Work out the finished part from the listing and answer in its coordinate system (mm). A direction names the side the tool comes from. Round coordinates to 2 decimals unless told otherwise and drop trailing zeros. Loops run counter-clockwise (first coordinate to the right, second up) from the corner with the lowest first, then second, coordinate; pieces in that order, holes last.
Autodesk Inventor part; units mm, degrees
ref_plane "YZ Plane" through (0, 0, 0) normal (1, 0, 0) x (0, 1, 0)
ref_plane "XZ Plane" through (0, 0, 0) normal (0, 1, 0) x (-1, 0, 0)
ref_plane "XY Plane" through (0, 0, 0) normal (0, 0, 1) x (1, 0, 0)
sketch "Sketch1" plane through (0, 0, 0) normal (0, 1, 0) x (-1, 0, 0)
  line L0 (65, -64) -> (-65, -64)
  line L1 (-65, -64) -> (-65, -45)
  line L2 (-65, 52) -> (65, 52)
  line L3 (65, 52) -> (65, -15)
  line L4 (94, -45) -> (65, -45)
  line L5 (65, -45) -> (65, -15) construction
  line L6 (65, -15) -> (94, -15)
  line L7 (94, -15) -> (94, -45)
  line L8 (-65, -45) -> (-94, -45)
  line L9 (-94, -45) -> (-94, -15)
  line L10 (-94, -15) -> (-65, -15)
  line L11 (-65, -15) -> (-65, -30) construction
  line L12 (94, -30) -> (-94, -30) construction
  line L13 (65, -45) -> (65, -64)
  line L14 (65, -15) -> (65, -45) construction
  line L15 (-65, -45) -> (-65, -15) construction
  line L16 (-65, -30) -> (-65, -45) construction
  line L17 (-65, -15) -> (-65, 52)
  point P0 (0, 0)
  point P1 (0, 52)
  dimension "d0" = 116
  dimension "d1" = 130
  dimension "d2" = 52
  dimension "d3" = 30
  dimension "d4" = 30
  dimension "d5" = 188
extrude "Extrusion1" add sketch "Sketch1" along normal blind 20
fillet "Fillet1" radius 10 4 edges at (65, 10, 52) (-65, 10, 52) (-65, 10, -64) (65, 10, -64)
sketch "Sketch2" plane through (0, 20, 0) normal (0, 1, 0) x (1, 0, 0)
  line L0 (65, 15) -> (94, 15)
  line L1 (94, 15) -> (94, 45)
  line L2 (94, 45) -> (65, 45)
  line L3 (94, 15) -> (94, 45)
  line L4 (65, 15) -> (94, 15)
  line L5 (94, 45) -> (76, 45)
  line L6 (76, 45) -> (76, 15)
  line L7 (76, 15) -> (94, 15)
  line L8 (94, 15) -> (94, 45)
  point P0 (0, 0)
  dimension "d9" = 18
extrude "Extrusion2" add sketch "Sketch2" along normal blind 38
fillet "Fillet2" radius 15 2 edges at (85, 58, -15) (85, 58, -45)
mirror "Mirror1" about plane through (0, 0, 0) normal (1, 0, 0) of "Extrusion2", "Fillet2"
sketch "Sketch3" plane through (94, 0, -15) normal (1, 0, 0) x (0, 0, -1)
  arc A0 (30, 43) -> (0, 43) centre (15, 43) ccw
  point P0 (-15, 0)
hole "Hole1" at (94, 43, -30) direction (-1, 0, 0) diameter 16 end through all
sketch "Sketch4" plane through (0, 20, 0) normal (0, 1, 0) x (1, 0, 0)
  line L0 (-55, -52) -> (55, -52)
  arc A0 (0, 24.1868) -> (0, -24.1868) centre (-28, 0) ccw
  line L1 (55, 64) -> (-55, 64)
  line L2 (0, 64) -> (0, -52) construction
  arc A1 (0, -24.1868) -> (0, 24.1868) centre (28, 0) ccw
  point P0 (0, 0)
  dimension "d20" = 74
  dimension "d21" = 56
extrude "Extrusion3" add sketch "Sketch4" along normal blind 6
sketch "Sketch5" plane through (0, 26, 0) normal (0, 1, 0) x (1, 0, 0)
  arc A0 (0, 24.1868) -> (0, -24.1868) centre (-28, 0) ccw
  point P0 (0, 0)
hole "Hole2" at (-28, 26, 0) direction (0, -1, 0) diameter 46 depth 15
sketch "Sketch6" plane through (0, 26, 0) normal (0, 1, 0) x (1, 0, 0)
  arc A0 (0, -24.1868) -> (0, 24.1868) centre (28, 0) ccw
  point P0 (0, 0)
  point P1 (28, 0)
hole "Hole3" at (28, 26, 0) direction (0, -1, 0) diameter 46 depth 15
sketch "Sketch7" plane through (65, 0, -15) normal (1, 0, 0) x (0, 0, -1)
  line L0 (-57, 0) -> (0, 0)
  line L1 (0, 0) -> (0, 20)
  line L2 (0, 0) -> (-32, 0)
  line L3 (-32, 0) -> (-32, 11)
  line L4 (-32, 11) -> (0, 11)
  line L5 (0, 11) -> (0, 0)
  point P0 (-15, 0)
  point P1 (0, 11)
  dimension "d38" = 32
  dimension "d39" = 11
extrude "Extrusion4" cut sketch "Sketch7" against normal through all
sketch "Sketch8" plane through (0, 20, 0) normal (0, 1, 0) x (1, 0, 0)
  arc A0 (65, 54) -> (55, 64) centre (55, 54) ccw
  arc A1 (-55, 64) -> (-65, 54) centre (-55, 54) ccw
  arc A2 (-65, 0) -> (0, -24.1868) centre (-28, 0) ccw
  line L0 (-65, 0) -> (-65, -42)
  arc A3 (-65, -42) -> (-55, -52) centre (-55, -42) ccw
  line L1 (-55, -52) -> (55, -52)
  arc A4 (55, -52) -> (65, -42) centre (55, -42) ccw
  line L2 (65, -42) -> (65, 0)
  arc A5 (0, -24.1868) -> (65, 0) centre (28, 0) ccw
  point P0 (0, 0)
hole "Hole4" at (-55, 20, -54) at (55, 20, -54) at (55, 20, 42) at (-55, 20, 42) direction (0, -1, 0) diameter 10 end through all
properties part number "Part023. Cylinder head" material "Steel, Carbon"
1. Determine the mould class of faces 4 (the face through (-85.1, 37.6, -24.1)), 5 (the face through (-1, 7, -15)), 6 (the face through (28, 11, 19)), 7 (the face through (84.9, 37.6, -24.1)) for opening direction Y: +Y half, -Y half, draft (parallel to the pull), parting line (faces both ways), or undercut.
Answer key:
face 4: undercut
face 5: draft
face 6: +Y half
face 7: undercut
2. Find section D-D (x = 16.5). Write down the section's boundary in (y, z), then the cut area to 3 significant figures.
Answer key:
outline: (0, -64) - (20, -64) - (20, -35.17) - (26, -35.17) - (26, -19.92) - (11, -19.92) - (11, -15) - (0, -15) - close; (0, 17) - (11, 17) - (11, 19.92) - (26, 19.92) - (26, 35.17) - (20, 35.17) - (20, 52) - (0, 52) - close
area: 1,790 mm2
3. Find section C-C (z = 6). Write down the section's boundary in (x, y), then the cut area to 3 significant figures.
Answer key:
outline: (-65, 11) - (-50.2, 11) - (-50.2, 26) - (-64.51, 26) - (-64.51, 20) - (-65, 20) - close; (-5.8, 11) - (5.8, 11) - (5.8, 26) - (-5.8, 26) - close; (50.2, 11) - (65, 11) - (65, 20) - (64.51, 20) - (64.51, 26) - (50.2, 26) - close
area: 612 mm2
4. Find section A-A (x = -28). Write down the section's boundary in (y, z), then the cut area to 3 significant figures.
Answer key:
outline: (0, -64) - (20, -64) - (20, -37) - (26, -37) - (26, -23) - (11, -23) - (11, -15) - (0, -15) - close; (0, 17) - (11, 17) - (11, 23) - (26, 23) - (26, 37) - (20, 37) - (20, 52) - (0, 52) - close
area: 1,720 mm2
5. Which of the six approach directions +Z, -Z, +X, -X, +Y, -Y give full straight-line access (tool end or side, diameter ignored) to faces 1 (the face through (-1, 26, -1)), 2 (the face through (-65, 10, -49)), 3 (the face through (5.196, 18.395, -2.994))?
Answer key:
face 1: +Z, -Z, +Y
face 2: -Z, -X, +Y, -Y
face 3: +Y
6. Given pin 1 (12 mm diameter, centred on x = -63.5, y = 11, fed in from +Z); pin 2 (21.5 mm diameter, centred on x = -44.5, y = 31.5, fed in from +Z); pin 3 (3 mm diameter, centred on y = 8.5, z = 2, fed in from +X); pin 4 (6 mm diameter, centred on y = 10.5, z = 0, fed in from +X), each flat-ended and moving along its own axis, determine where each tip first touches the part or whether it passes through.
Answer key:
pin 1: stops at z = 51.68
pin 2: stops at z = 36.28
pin 3: passes through
pin 4: stops at x = 65
7. Consider probe 1 along X at (y, z) = (12, -54); probe 2 along Z at (x, y) = (-55, 6.25); probe 3 along X at (y, z) = (50, -41). Determine where each line is inside the solid, lowest interval first.
Answer key:
probe 1: x = -65 to -60, -50 to 50, 60 to 65
probe 2: z = -64 to -59, -49 to -15, 17 to 37, 47 to 52
probe 3: x = -94 to -76, 76 to 94
